from build123d import *

# Parameters (mm, degrees)
F0_W     = 1168.4
F0_H     = 742.95
F1_DEPTH = 19.05
F2_W     = 19.05
F2_H     = 742.95
F3_DEPTH = 50.8
F4_W     = 19.05
F4_H     = 314.325
F5_DEPTH = 263.525
F6_W     = 19.05
F6_H     = 314.325
F7_DEPTH = 263.525
F8_DEPTH = 152.4


with BuildPart() as f1:
    # F0 (on Front) → F1 (new body)
    with BuildSketch(Plane.XZ):
        Rectangle(F0_W, F0_H)
    extrude(amount=F1_DEPTH)

    # F2 (on face) → F3 (join)
    with BuildSketch(Plane(origin=(0, 0, 0), x_dir=(-1, 0, 0), z_dir=(0, 1, 0))):
        with Locations((-574.675, 0)):
            Rectangle(F2_W, F2_H)
        with Locations((574.675, 0)):
            Rectangle(F2_W, F2_H)
    extrude(amount=F3_DEPTH)

    # F4 (on face) → F5 (join)
    with BuildSketch(Plane(origin=(0, 50.8, 0), x_dir=(-1, 0, 0), z_dir=(0, 1, 0))):
        with Locations((-574.675, 214.3125)):
            Rectangle(F4_W, F4_H)
    extrude(amount=F5_DEPTH)

    # F6 (on face) → F7 (join)
    with BuildSketch(Plane(origin=(0, 50.8, 0), x_dir=(-1, 0, 0), z_dir=(0, 1, 0))):
        with Locations((574.675, 214.3125)):
            Rectangle(F6_W, F6_H)
    extrude(amount=F7_DEPTH)

    # F8 (add): a face of the model
    f8_faces = [f1.faces().sort_by_distance(p)[0] for p in [
        (0, -6.731, -371.475),
    ]]
    extrude(f8_faces, amount=F8_DEPTH)


solid = f1.part
Could you check a few things on this model? Use its own coordinates, in mm. A direction names the side the tool comes from. Round coordinates to 2 decimals unless told otherwise and drop trailing zeros. Write each loop counter-clockwise with the first axis right and the second up, starting at its lowest first coordinate (ties: lowest second). Pieces come first, ordered by that corner, then holes. Notation, with made-up numbers: (36, -29.5) - (45, -29.5) arc R34 ccw to (45, 6.5) - close; hole circle Ø4 at (39, 68). An arc over 180 degrees is marked (long way). Use a Markdown table: item, result.
Q1. Thinking about a two-plate mould opening in X: for faces 3 (the flat face through (46, -5, -523.875)), 4 (the flat face through (584.2, 108, 129)), 5 (the flat face through (-8, 0, -70)), which applies, released by +X, released by -X, zero draft, split by the parting line, or undercut?
Output values:
| item | result |
|---|---|
| face 3 | zero draft |
| face 4 | released by +X |
| face 5 | undercut |
Q2. For faces 1 (the flat face through (-565.15, 120, 129)), 2 (the flat face through (176, -1, 371.475)), which set-ups out of +Z, -Z, +X, -X, +Y, -Y let a thin tool reach every point of the face, with its end or its side?
Output values:
| item | result |
|---|---|
| face 1 | +Z, -Z, +Y |
| face 2 | +Z, +X, -X, +Y, -Y |
Q3. I want a section at B-B (z = -445.5). List the corners of the cut face in (x, y) for me.
Output values:
| item | result |
|---|---|
| outline | (-584.2, -19.05) - (584.2, -19.05) - (584.2, 50.8) - (565.15, 50.8) - (565.15, 0) - (-565.15, 0) - (-565.15, 50.8) - (-584.2, 50.8) - close |
Q4. I want a section at A-A (y = 178). List the corners of the cut face in (x, z) for me (3 decimals), plus the area to 3 significant figures.
Output values:
| item | result |
|---|---|
| outline | (-584.2, 57.15) - (-565.15, 57.15) - (-565.15, 371.475) - (-584.2, 371.475) - close; (565.15, 57.15) - (584.2, 57.15) - (584.2, 371.475) - (565.15, 371.475) - close |
| area | 12,000 mm2 |
Q5. Please list where these lines run through material, in increasing order: L1, parallel to X at y = 148, z = 287; L2, parallel to Y at x = -346, z = 130.
Output values:
| item | result |
|---|---|
| L1 | -584.2 to -565.15, 565.15 to 584.2 |
| L2 | -19.05 to 0 |
Q6. For pin 1 (4 mm diameter, centred on x = -36.5, z = -39, fed in from +Y); pin 2 (5.5 mm diameter, centred on x = 571, y = 189, fed in from -Z); pin 3 (9.5 mm diameter, centred on x = -577, z = -303.5, fed in from +Y), each with a flat end and sliding along its axis, tell me the tip position at first contact or that it passes through.
Output values:
| item | result |
|---|---|
| pin 1 | y = 0 |
| pin 2 | z = 57.15 |
| pin 3 | y = 50.8 |
Q7. I want a section at D-D (z = 159.5). List the corners of the cut face in (x, y) for me (3 decimals).
Output values:
| item | result |
|---|---|
| outline | (-584.2, -19.05) - (584.2, -19.05) - (584.2, 314.325) - (565.15, 314.325) - (565.15, 0) - (-565.15, 0) - (-565.15, 314.325) - (-584.2, 314.325) - close |
Q8. I want a section at C-C (x = -82). List the corners of the cut face in (y, z) for me (3 decimals), plus the area to 3 significant figures.
Output values:
| item | result |
|---|---|
| outline | (-19.05, -523.875) - (0, -523.875) - (0, 371.475) - (-19.05, 371.475) - close |
| area | 17,100 mm2 |
